Work out the finished part from the listing and answer in its coordinate system (mm). Round coordinates to 2 decimals unless told otherwise and drop trailing zeros. Loops run counter-clockwise (first coordinate to the right, second up) from the corner with the lowest first, then second, coordinate; pieces in that order, holes last. Notation, with made-up numbers: M 35,61 L 42,61 A19 ccw 42,75 Z; hole C 19.25,62 d2. An arc over 180 degrees is marked long. One line per item, written item: value.
```python
from build123d import *

# Parameters (mm, degrees)
MAIN_DEPTH               = 5.13
M3_CLEARANCE_HOLE1_D     = 3.2
M3_CLEARANCE_HOLE1_DEPTH = 5.13
SKETCH4_W                = 16.6
SKETCH4_H                = 5.13
TOP_TABS_DEPTH           = 5.13
T_SLOT_DEPTH             = 1
T_SLOT_DEPTH_BACK        = 6.13


with BuildPart() as part:
    # Sketch1 → Main (new body)
    with BuildSketch(Plane.XY):
        with BuildLine():
            Line((-54.096109727, 17.496253248), (44.263890273, 17.496253248))
            Line((44.263890273, 17.496253248), (44.263890273, -10.503746752))
            ThreePointArc((44.263890273, -10.503746752), (43.970997054, -11.210853533), (43.263890273, -11.503746752))
            Line((43.263890273, -11.503746752), (-53.096109727, -11.503746752))
            ThreePointArc((-53.096109727, -11.503746752), (-53.803216508, -11.210853533), (-54.096109727, -10.503746752))
            Line((-54.096109727, -10.503746752), (-54.096109727, 17.496253248))
        make_face()
    extrude(amount=MAIN_DEPTH)

    # M3 Clearance Hole1
    with Locations(Plane.XY.offset(5.13)):
        with Locations((-44.530109727, 3.996253248), (34.697890273, 3.996253248)):
            Hole(M3_CLEARANCE_HOLE1_D / 2, depth=M3_CLEARANCE_HOLE1_DEPTH)

    # Sketch4 → top tabs (add)
    with BuildSketch(Plane(origin=(0, 17.496253248, 0), x_dir=(1, 0, 0), z_dir=(0, 1, 0))):
        with Locations((11.683890273, -2.565)):
            Rectangle(SKETCH4_W, SKETCH4_H)
        with Locations((-21.516109727, -2.565)):
            Rectangle(SKETCH4_W, SKETCH4_H)
    extrude(amount=TOP_TABS_DEPTH)

    # Sketch5 → t-slot (cut, two sides)
    with BuildSketch(Plane.XY.offset(5.13)) as t_slot_sk:
        Polygon((-6.414608826, 144.274852992), (-6.414608826, 17.496253838), (-6.414608826, 13.501253838), (-7.773611823, 13.501254105), (-7.77361225, 11.334254105), (-6.41461225, 11.334253838), (-6.414613471, 5.127253838), (-3.417613471, 5.127253248), (-3.41761225, 11.334253248), (-2.05861225, 11.334252981), (-2.058611823, 13.501252981), (-3.417610628, 13.501253248), (-3.417610628, 17.496253248), (-3.417610628, 144.274852403), (-3.41756075, 397.832050712), (-6.414558948, 397.832051301), align=None)
    extrude(amount=T_SLOT_DEPTH, mode=Mode.SUBTRACT)
    extrude(t_slot_sk.sketch, amount=-T_SLOT_DEPTH_BACK, mode=Mode.SUBTRACT)


solid = part.part
```
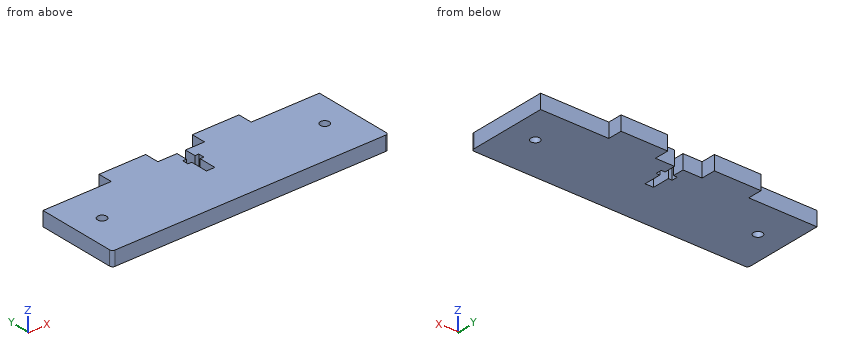
1) Find section B-B (z = 3.25). Give the vertices of the cut face in (x, y).
Check values:
outline: M -54.1,-10.5 A1 ccw -53.1,-11.5 L 43.26,-11.5 A1 ccw 44.26,-10.5 L 44.26,17.5 L 19.98,17.5 L 19.98,22.63 L 3.38,22.63 L 3.38,17.5 L -3.42,17.5 L -3.42,13.5 L -2.06,13.5 L -2.06,11.33 L -3.42,11.33 L -3.42,5.13 L -6.41,5.13 L -6.41,11.33 L -7.77,11.33 L -7.77,13.5 L -6.41,13.5 L -6.41,17.5 L -13.22,17.5 L -13.22,22.63 L -29.82,22.63 L -29.82,17.5 L -54.1,17.5 Z; hole C -44.53,4 d3.2; hole C 34.7,4 d3.2
2) Find section C-C (y = 20). Give the vertices of the cut face in (x, z).
Check values:
outline: M -29.82,0 L -13.22,0 L -13.22,5.13 L -29.82,5.13 Z; M 3.38,0 L 19.98,0 L 19.98,5.13 L 3.38,5.13 Z
3) Find the intervals of material crossed by probe 1 along X at (y, z) = (12.5, 2.2); probe 2 along X at (y, z) = (15, 0.5); probe 3 along Y at (x, z) = (-39.5, 1.35), in increasing order. Write a range as from..to.
Check values:
probe 1: -54.1..-7.77, -2.06..44.26
probe 2: -54.1..-6.41, -3.42..44.26
probe 3: -11.5..17.5
4) Each of these flat-tipped pins is pushed along its axis until it touches: pin 1 (2.5 mm diameter, centred on x = -40, z = 3.5, fed in from +Y); pin 2 (1.5 mm diameter, centred on x = -4.5, z = 1.5, fed in from +Y); pin 3 (2.5 mm diameter, centred on y = 19.5, z = 3.5, fed in from -X). Where does it stop, or does it pass through?
Check values:
pin 1: y = 17.5
pin 2: y = 5.13
pin 3: x = -29.82
5) Find section D-D (x = -31). Give the vertices of the cut face in (y, z), then the cut area to 3 significant figures.
Check values:
outline: M -11.5,0 L 17.5,0 L 17.5,5.13 L -11.5,5.13 Z
area: 149 mm2
6) Find section A-A (y = 8). Give the vertices of the cut face in (x, z), then the cut area to 3 significant figures.
Check values:
outline: M -54.1,0 L -6.41,0 L -6.41,5.13 L -54.1,5.13 Z; M -3.42,0 L 44.26,0 L 44.26,5.13 L -3.42,5.13 Z
area: 489 mm2
